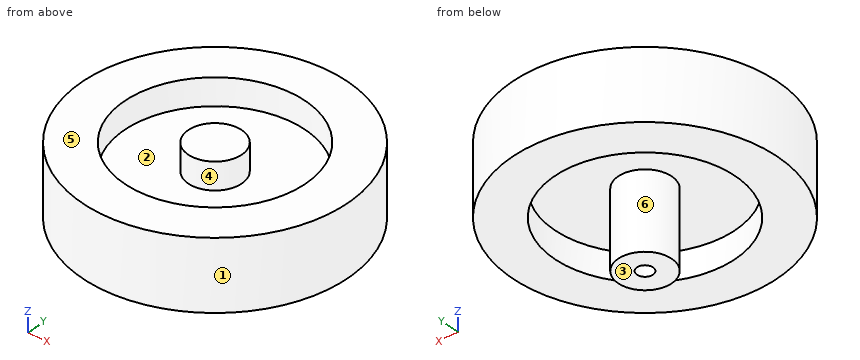
from build123d import *

# Parameters (mm, degrees)
ESQUISSE1_R             = 49.5
BOSS_EXTRU_2_DEPTH      = 13
ESQUISSE5_R             = 33.75
ESQUISSE5_R_2           = 10
ENL_V_MAT_EXTRU_1_DEPTH = 10
ESQUISSE12_R            = 10
BOSS_EXTRU_3_DEPTH      = 18.5
ESQUISSE13_R            = 3
ENL_V_MAT_EXTRU_2_DEPTH = 10


with BuildPart() as part:
    # Esquisse1 → Boss.-Extru.2 (new body)
    with BuildSketch(Plane.XY):
        with Locations(Location((0, 0, 0), (0, 0, 180))):
            Circle(ESQUISSE1_R)
    extrude(amount=BOSS_EXTRU_2_DEPTH)

    # Esquisse5 → Enlèv. mat.-Extru.1 (cut)
    with BuildSketch(Plane.XY.offset(13)):
        Circle(ESQUISSE5_R)
        Circle(ESQUISSE5_R_2, mode=Mode.SUBTRACT)
    extrude(amount=-ENL_V_MAT_EXTRU_1_DEPTH, mode=Mode.SUBTRACT)

    # Symétrie6: part across plane


with BuildPart() as part_1:
    add(part.part)
    add(part.part.mirror(Plane.XY))

    # Esquisse12 → Boss.-Extru.3 (add)
    with BuildSketch(Plane(origin=(0, 0, -13), x_dir=(-1, 0, 0), z_dir=(0, 0, -1))):
        with Locations(Location((0, 0, 0), (0, 0, 180))):
            Circle(ESQUISSE12_R)
    extrude(amount=BOSS_EXTRU_3_DEPTH)

    # Esquisse13 → Enlèv. mat.-Extru.2 (cut)
    with BuildSketch(Plane(origin=(0, 0, -31.5), x_dir=(-1, 0, 0), z_dir=(0, 0, -1))):
        Circle(ESQUISSE13_R)
    extrude(amount=-ENL_V_MAT_EXTRU_2_DEPTH, mode=Mode.SUBTRACT)


solid = part_1.part
Verification items for the finished model (mm, model axes). Face numbers are marked on the shaded views. A direction names the side the tool comes from. Give positions to 0.01 mm unless a question says otherwise; leave off trailing zeros. Loops run counter-clockwise (first coordinate to the right, second up) from the corner with the lowest first, then second, coordinate; pieces in that order, holes last.
1. Material ranges on probe 1 along Y at (x, z) = (0, -9.5); probe 2 along Y at (x, z) = (0, -28); probe 3 along Z at (x, y) = (11.5, -16), recorded low to high.
Derived:
probe 1: y = -49.5 to -33.75, -10 to 10, 33.75 to 49.5
probe 2: y = -10 to -3, 3 to 10
probe 3: z = -3 to 3
2. Go/stop test with flat-tipped pins: P1, Ø12, axis at x = -29.5, y = 27, coming from the -Z side; P2, Ø2, axis at x = 29.5, y = -8.5, coming from the +Z side; P3, Ø1.5, axis at y = -24.5, z = 0.5, coming from the -X side. Record where each tip stops, or that it passes through.
Derived:
P1: stops at z = -13
P2: stops at z = 3
P3: stops at x = -43.43
3. Cross-section at A-A on z = 7.5. Record the cut outline in (x, y), and give its area (3 significant figures).
Derived:
outline: circle Ø99 at (0, 0); circle Ø20 at (0, 0); hole circle Ø67.5 at (0, 0)
area: 4,430 mm2
4. Cross-section at B-B on x = 0. Record the cut outline in (y, z), and give its area (3 significant figures).
Derived:
outline: (-49.5, -13) - (-33.75, -13) - (-33.75, -3) - (-10, -3) - (-10, -31.5) - (-3, -31.5) - (-3, -21.5) - (3, -21.5) - (3, -31.5) - (10, -31.5) - (10, -3) - (33.75, -3) - (33.75, -13) - (49.5, -13) - (49.5, 13) - (33.75, 13) - (33.75, 3) - (10, 3) - (10, 13) - (-10, 13) - (-10, 3) - (-33.75, 3) - (-33.75, 13) - (-49.5, 13) - close
area: 1,930 mm2
5. Release check for a two-part mould opening along X. For the marked faces 1, 2 and 3 record: +X half, -X half, draft (parallel to the pull), parting line (faces both ways), or undercut.
Derived:
face 1: parting line
face 2: undercut
face 3: draft
6. Tool access check on the marked faces 4, 5 and 6. Record the directions out of +Z, -Z, +X, -X, +Y, -Y that give a thin tool (end or side, any length) a straight path to the whole face; none if there is none.
Derived:
face 4: +Z
face 5: +Z, +X, -X, +Y, -Y
face 6: -Z
7. Cross-section at D-D on z = -1.5. Record the cut outline in (x, y), and give its area (3 significant figures).
Derived:
outline: circle Ø99 at (0, 0)
area: 7,700 mm2
